```python
from build123d import *

# Parameters (mm, degrees)
SZKIC1_W                    = 60
SZKIC1_H                    = 8
DODANIE_WYCI_GNI_CIE1_DEPTH = 3
ZAOKR_GLENIE1_R             = 4
SZKIC2_R                    = 1.5
WYTNIJ_WYCI_GNI_CIE1_DEPTH  = 3
DODANIE_WYCI_GNI_CIE2_DEPTH = 3
SFAZOWANIE1_SIZE            = 4
SFAZOWANIE1_SIZE_2          = 3.0142162
WYTNIJ_WYCI_GNI_CIE2_DEPTH  = 3


# Some blends are built 0.0001 mm under size
with BuildPart() as part:
    # Szkic1 → Dodanie-wyciągnięcie1 (new body)
    with BuildSketch(Plane.XY):
        with Locations((30, 4)):
            Rectangle(SZKIC1_W, SZKIC1_H)
    extrude(amount=DODANIE_WYCI_GNI_CIE1_DEPTH)

    # Zaokrąglenie1
    zaokr_glenie1_edges = [part.edges().sort_by_distance(p)[0] for p in [
        (60, 0, 1.5),
        (60, 8, 1.5),
        (0, 8, 1.5),
        (0, 0, 1.5),
    ]]
    fillet(zaokr_glenie1_edges, radius=ZAOKR_GLENIE1_R - 0.0001)  # a hair under: the kernel refuses the full size

    # Szkic2 → Wytnij-wyciągnięcie1 (cut)
    with BuildSketch(Plane.XY.offset(3)):
        with Locations((4, 4)):
            Circle(SZKIC2_R)
        with Locations((56, 4)):
            Circle(SZKIC2_R)
    extrude(amount=-WYTNIJ_WYCI_GNI_CIE1_DEPTH, mode=Mode.SUBTRACT)

    # Szkic3 → Dodanie-wyciągnięcie2 (add)
    with BuildSketch(Plane.XY.offset(3)):
        Polygon((5.2, 8), (17, 0), (22, 0), (22, 8), align=None)
    extrude(amount=DODANIE_WYCI_GNI_CIE2_DEPTH)

    # Sfazowanie1
    # the kernel refuses this chamfer: 4, 3.0142162 mm, written as the material it adds along each edge
    with BuildSketch(Plane(origin=(22, 0, 3), x_dir=(0.9997280272590686, 0, -0.023321052992758322), z_dir=(0, 1, 0))) as sfazowanie1_piece_1_section:
        Polygon((SFAZOWANIE1_SIZE * 0.999728027259, -SFAZOWANIE1_SIZE * 0.0233210529928), (-SFAZOWANIE1_SIZE_2 * 0.0233210529959, -SFAZOWANIE1_SIZE_2 * 0.999728027395), (0, 0), align=None)
    sfazowanie1_piece_1 = extrude(amount=8, mode=Mode.PRIVATE)
    sfazowanie1_piece_1 = split(sfazowanie1_piece_1, bisect_by=Plane(origin=(23.333090008, 4, 6), z_dir=(0, 0, -1)), keep=Keep.TOP, mode=Mode.PRIVATE)
    add(sfazowanie1_piece_1)

    # Szkic4 → Wytnij-wyciągnięcie2 (cut)
    with BuildSketch(Plane.XY.offset(6)):
        Polygon((5.2, 8), (11.1, 4), (11.1, 8), align=None)
    extrude(amount=-WYTNIJ_WYCI_GNI_CIE2_DEPTH, mode=Mode.SUBTRACT)


solid = part.part
```
Verification items for the finished model (mm, model axes). A direction names the side the tool comes from. Coordinates: 2 decimals unless noted, no trailing zeros. Loops run counter-clockwise (first coordinate to the right, second up) from the corner with the lowest first, then second, coordinate; pieces in that order, holes last. Notation, with made-up numbers: (-35, -22.75) -> (-17, -22.75) arc R18 cw to (-17, -1.75) -> close; hole circle Ø9 at (43, -8). An arc over 180 degrees is marked (long way). Answer in a Markdown table with one row per item. Add a question column.
1. Section check A-A, the plane z = 1.35. Give the number of separate pieces and of enclosed holes in the cut face, then the cut area to 3 significant figures.
2. Section check D-D, the plane x = 46.5. Enter the section's corners in (y, z).
3. Draft check along Y on faces 1 (the face through (24.037, 3.944, 4.479)), 2 (the face through (57.43, 4.45, 1.52)), 3 (the face through (30, 0, 2)). Enter one of: +Y half, -Y half, draft (parallel to the pull), parting line (faces both ways), or undercut.
4. Depth check by flat-ended pin: P1, Ø4, axis at x = 4, y = 4, coming from the +Z side; P2, Ø1, axis at y = 6.5, z = 3, coming from the -X side; P3, Ø1.5, axis at y = 5.5, z = 5, coming from the -X side. Enter the tip coordinate at first touch or a pass-through.
5. Access from +Z, -Z, +X, -X, +Y, -Y to the whole of each face (thin tool, end or side, straight path). Record for faces 4 (the face through (43, 4, 3)), 5 (the face through (30, 8, 2)), 6 (the face through (11.1, 6, 5)), 7 (the face through (6, 4, 3)).
6. Material ranges on probe 1 along Y at (x, z) = (4, 1.6); probe 2 along X at (y, z) = (5.25, 0.7); probe 3 along Z at (x, y) = (42.5, 2.5), recorded low to high. Write a range as [from, to].
7. Section check C-C, the plane y = 7.5. Enter the section's corners in (x, z), then the cut area to 3 significant figures.
8. Section check B-B, the plane y = 5. Enter the section's corners in (x, z), then the cut area to 3 significant figures.
Derived:
| question | item | result |
|---|---|---|
| 1 | separate pieces | 1 |
| 1 | enclosed holes | 2 |
| 1 | area | 452 mm² |
| 2 | outline | (0, 0) -> (8, 0) -> (8, 3) -> (0, 3) -> close |
| 3 | face 1 | draft |
| 3 | face 2 | undercut |
| 3 | face 3 | -Y half |
| 4 | P1 | stops at z = 3 |
| 4 | P2 | stops at x = 0.54 |
| 4 | P3 | stops at x = 11.1 |
| 5 | face 4 | +Z, +X, +Y, -Y |
| 5 | face 5 | +Z, -Z, +X, -X, +Y |
| 5 | face 6 | +Z, -X, +Y, -Y |
| 5 | face 7 | +Z, -X, -Y |
| 6 | probe 1 | y = [0, 2.5], [5.5, 8] |
| 6 | probe 2 | x = [0.2, 3.17], [4.83, 55.17], [56.83, 59.8] |
| 6 | probe 3 | z = [0, 3] |
| 7 | outline | (2.06, 0) -> (57.94, 0) -> (57.94, 3) -> (26, 3) -> (22.02, 6) -> (11.1, 6) -> (11.1, 3) -> (2.06, 3) -> close |
| 7 | area | 206 mm² |
| 8 | outline | (0.13, 0) -> (2.88, 0) -> (2.88, 3) -> (0.13, 3) -> close; (5.12, 0) -> (54.88, 0) -> (54.88, 3) -> (26, 3) -> (22.02, 6) -> (11.1, 6) -> (11.1, 3) -> (5.12, 3) -> close; (57.12, 0) -> (59.87, 0) -> (59.87, 3) -> (57.12, 3) -> close |
| 8 | area | 205 mm² |
